Source: CAD feature listing. Evaluate the final solid. Frame: model axes, mm. A direction names the side the tool comes from. Give positions to 0.01 mm unless a question says otherwise; leave off trailing zeros. Loops run counter-clockwise (first coordinate to the right, second up) from the corner with the lowest first, then second, coordinate; pieces in that order, holes last. Notation, with made-up numbers: (2.5, -38) -> (38.5, -38) arc R9 cw to (38.5, -28) -> close; hole circle Ø9 at (50.5, 3.25). An arc over 180 degrees is marked (long way). Return JSON: item names as keys, results as strings. Group by question number.
(1) Access query for faces 4 (the face through (20, 0, 100)), 5 (the face through (-1, 27, 80)), 6 (the face through (0, -20, 95)), 7 (the face through (-20, 0, 100)). Directions: +Z, -Z, +X, -X, +Y, -Y. A direction counts if a zero-diameter tool reaches every point of the face in a straight line with its end or side. Return the directions, or none.
(2) Draft query along X for faces 1 (the face through (0, 20, 95)), 2 (the face through (-40, -1, 39)), 3 (the face through (8.37, -0.28, 101.68)). Return one class per face: released by +X, released by -X, zero draft, split by the parting line, or undercut.
(3) Cut plane D-D on x = -22. Return loops of the section in (y, z).
(4) Pin query (flat end, axial travel): pin 1 (20 mm diameter, centred on x = 4.5, z = 97, fed in from +Y); pin 2 (3 mm diameter, centred on x = 15.5, y = 30, fed in from +Z); pin 3 (1 mm diameter, centred on x = 20, y = -18, fed in from -Z); pin 4 (12 mm diameter, centred on y = -7.5, z = 105.5, fed in from -X). Return the tip coordinate at first contact, or that it passes through.
(5) Cut plane C-C on y = 16. Return loops of the section in (x, z), then the cut area to 3 significant figures.
(6) Ray query, line 1 (Z direction, x = 10, y = -7); line 2 (Z direction, x = -18, y = -24.5); line 3 (Y direction, x = -4, z = 99.5). Return the intervals inside material, ascending. Write a range as from..to.
(7) Cut plane B-B on x = -10. Return loops of the section in (y, z).
(8) Cut plane A-A on z = 109. Return loops of the section in (x, y), then the cut area to 3 significant figures.
```python
from build123d import *

# Parameters (mm, degrees)
F0_W     = 80
F0_H     = 80
F1_DEPTH = 80
F2_W     = 40
F2_H     = 40
F3_DEPTH = 40
F4_R     = 7.5
F5_DEPTH = 40
F6_R     = 7.5
F7_DEPTH = 40


with BuildPart() as f1:
    # F0 (on Top) → F1 (new body)
    with BuildSketch(Plane.XY):
        Rectangle(F0_W, F0_H)
    extrude(amount=F1_DEPTH)

    # F2 (on face) → F3 (join)
    with BuildSketch(Plane.XY.offset(80)):
        Rectangle(F2_W, F2_H)
    extrude(amount=F3_DEPTH)

    # F4 (on face) → F5 (cut)
    with BuildSketch(Plane.XZ.offset(20)):
        with Locations((-10, 109)):
            Circle(F4_R)
    extrude(amount=-F5_DEPTH, mode=Mode.SUBTRACT)

    # F6 (on face) → F7 (cut)
    with BuildSketch(Plane.XZ.offset(20)):
        with Locations((10, 109)):
            Circle(F6_R)
    extrude(amount=-F7_DEPTH, mode=Mode.SUBTRACT)


solid = f1.part
```
Answers:
{
 "1": {"face 4": "+Z, +X, +Y, -Y", "face 5": "+Z", "face 6": "+Z, +X, -X, -Y", "face 7": "+Z, -X, +Y, -Y"},
 "2": {"face 1": "zero draft", "face 2": "released by -X", "face 3": "undercut"},
 "3": {"outline": "(-40, 0) -> (40, 0) -> (40, 80) -> (-40, 80) -> close"},
 "4": {"pin 1": "y = 20", "pin 2": "z = 80", "pin 3": "z = 0", "pin 4": "x = -20"},
 "5": {"outline": "(-40, 0) -> (40, 0) -> (40, 80) -> (20, 80) -> (20, 120) -> (-20, 120) -> (-20, 80) -> (-40, 80) -> close; hole circle Ø15 at (-10, 109); hole circle Ø15 at (10, 109)", "area": "7,650 mm²"},
 "6": {"line 1": "0..101.5, 116.5..120", "line 2": "0..80", "line 3": "-20..20"},
 "7": {"outline": "(-40, 0) -> (40, 0) -> (40, 80) -> (20, 80) -> (20, 101.5) -> (-20, 101.5) -> (-20, 80) -> (-40, 80) -> close; (-20, 116.5) -> (20, 116.5) -> (20, 120) -> (-20, 120) -> close"},
 "8": {"outline": "(-20, -20) -> (-17.5, -20) -> (-17.5, 20) -> (-20, 20) -> close; (-2.5, -20) -> (2.5, -20) -> (2.5, 20) -> (-2.5, 20) -> close; (17.5, -20) -> (20, -20) -> (20, 20) -> (17.5, 20) -> close", "area": "400 mm²"}
}
